Source: CAD feature listing. Evaluate the final solid. Frame: model axes, mm. Round coordinates to 2 decimals unless told otherwise and drop trailing zeros. Write each loop counter-clockwise with the first axis right and the second up, starting at its lowest first coordinate (ties: lowest second). Pieces come first, ordered by that corner, then holes. Notation, with made-up numbers: M -13.5,72 L 31.5,72 A15 cw 31.5,77 Z; hole C 23,22.25 d4. An arc over 180 degrees is marked long. Answer in a Markdown table with one row per item.
from build123d import *

# Parameters (mm, degrees)
SKETCH1_R           = 2.5
SKETCH1_R_2         = 1.6
BOSS_EXTRUDE1_DEPTH = 1000
SKETCH2_R           = 2.5
SKETCH2_R_2         = 1.6
BOSS_EXTRUDE2_DEPTH = 500
SKETCH3_R           = 2.5
SKETCH3_R_2         = 1.6
BOSS_EXTRUDE3_DEPTH = 500


with BuildPart() as part:
    # Sketch1 → Boss-Extrude1 (new body)
    with BuildSketch(Plane.XY):
        Circle(SKETCH1_R)
        Circle(SKETCH1_R_2, mode=Mode.SUBTRACT)
    extrude(amount=BOSS_EXTRUDE1_DEPTH)

    # Sketch2 → Boss-Extrude2 (add)
    with BuildSketch(Plane.XY.offset(1000)):
        Circle(SKETCH2_R)
        Circle(SKETCH2_R_2, mode=Mode.SUBTRACT)
    extrude(amount=BOSS_EXTRUDE2_DEPTH)

    # Sketch3 → Boss-Extrude3 (add)
    with BuildSketch(Plane.XY.offset(1500)):
        Circle(SKETCH3_R)
        Circle(SKETCH3_R_2, mode=Mode.SUBTRACT)
    extrude(amount=BOSS_EXTRUDE3_DEPTH)


solid = part.part
Q1. Section C-C (z = 1342.5). Return loops of the section in (x, y).
Solutions:
| item | result |
|---|---|
| outline | C 0,0 d5; hole C 0,0 d3.2 |
Q2. Section A-A (x = 0). Return loops of the section in (y, z), and give its area (3 significant figures).
Solutions:
| item | result |
|---|---|
| outline | M -2.5,0 L -1.6,0 L -1.6,2000 L -2.5,2000 Z; M 1.6,0 L 2.5,0 L 2.5,2000 L 1.6,2000 Z |
| area | 3,600 mm2 |
Q3. Material intervals for probe 1 along Y at (x, z) = (-0.8, 1235); probe 2 along Y at (x, z) = (-0.5, 1489); probe 3 along X at (y, z) = (0.25, 1903.5), sorted ascending.
Solutions:
| item | result |
|---|---|
| probe 1 | y = -2.37 to -1.39, 1.39 to 2.37 |
| probe 2 | y = -2.45 to -1.52, 1.52 to 2.45 |
| probe 3 | x = -2.49 to -1.58, 1.58 to 2.49 |
